from build123d import *

# Parameters (mm, degrees)
ESBO_O1_R             = 75
ESBO_O1_R_2           = 8.5
EXTRUS_O1_DEPTH       = 3.35
ESBO_O2_R             = 24.25
CORTE_EXTRUS_O1_DEPTH = 1
CORTE_EXTRUS_O3_DEPTH = 10
LPATTERN3_COUNT       = 2
LPATTERN3_PITCH       = 28
FILETE1_R             = 2


with BuildPart() as part:
    # Esboço1 → Extrusão1 (new body)
    with BuildSketch(Plane.XY):
        Circle(ESBO_O1_R)
        Circle(ESBO_O1_R_2, mode=Mode.SUBTRACT)
    extrude(amount=EXTRUS_O1_DEPTH)

    # Esboço2 → Corte-extrusão1 (cut)
    with BuildSketch(Plane(origin=(0, 0, 0), x_dir=(-1, 0, 0), z_dir=(0, 0, -1))):
        Circle(ESBO_O2_R)
    extrude(amount=-CORTE_EXTRUS_O1_DEPTH, mode=Mode.SUBTRACT)

    # Esboço6 → Corte-extrusão3 (cut)
    with BuildSketch(Plane(origin=(0, 0, 0), x_dir=(-1, 0, 0), z_dir=(0, 0, -1))):
        with BuildLine():
            Line((-5, 25.5), (5, 25.5))
            ThreePointArc((5, 25.5), (7.5, 28), (5, 30.5))
            Line((5, 30.5), (-5, 30.5))
            ThreePointArc((-5, 30.5), (-7.5, 28), (-5, 25.5))
        make_face()
    extrude(amount=-CORTE_EXTRUS_O3_DEPTH, mode=Mode.SUBTRACT)

    # Esboço8 → Escareado para SFHCS M63 (revolve, cut)
    with BuildSketch(Plane(origin=(17.5, 33.25, 0), x_dir=(0, 1, 0), z_dir=(1, 0, 0))):
        Polygon((0, 0), (0, 3.35), (3.3, 3.35), (3.3, 3.42), (6.72, 0), align=None)
    escareado_para_sfhcs_m63 = revolve(axis=Axis((17.5, 33.25, -6.35), (0, 0, 1)), mode=Mode.SUBTRACT)

    # LPattern3: Escareado para SFHCS M63 ×2
    with Locations(*[(i * LPATTERN3_PITCH, 0, 0) for i in range(1, LPATTERN3_COUNT)]):
        add(escareado_para_sfhcs_m63, mode=Mode.SUBTRACT)

    # Filete1
    filete1_edges = [part.edges().sort_by_distance(p)[0] for p in [
        (-75, 0, 0),
    ]]
    fillet(filete1_edges, radius=FILETE1_R)


solid = part.part
Work out the finished part from the listing and answer in its coordinate system (mm). A direction names the side the tool comes from. Give positions to 0.01 mm unless a question says otherwise; leave off trailing zeros. Order: outer loops, then holes, each group sorted by start corner. A loop starts at its lowest first (then second) coordinate and runs counter-clockwise, first axis right, second up. Notation, with made-up numbers: (-23.75, -18.75) -> (-7.75, -18.75) arc R19 cw to (-7.75, -14.75) -> close; hole circle Ø6 at (62.25, -21.5). An arc over 180 degrees is marked (long way). Answer as a JSON object with one key per item and string values. Group by question number.
1. Section A-A on x = 0 is taken. Determine the outline of the cut face in (y, z), plus the area to 3 significant figures.
2. The mould has two halves that part along Y. Classify faces 1 (the flat face through (-10, 0, 1)), 2 (the cylindrical face through (-9.764, 74.362, 2.666)), 3 (the flat face through (-1, -31, 0)): released by +Y, released by -Y, zero draft, split by the parting line, or undercut.
3. A tool of negligible diameter and unlimited length cuts with its end or side. For faces 4 (the flat face through (0, 25.5, 2)), 5 (the cylindrical face through (-11.19, -21.514, 0.493)), 6 (the flat face through (-1, -16, 3.35)), from which of +Z, -Z, +X, -X, +Y, -Y can it reach the whole face along a straight path? Write none if from no direction.
4. Section B-B on y = 0 is taken. Determine the outline of the cut face in (x, z).
5. Flat-ended cylindrical pins translate along their axes: pin 1 Ø4 at (x, y) = (-26, 37) entering from -Z; pin 2 Ø1 at (x, z) = (31, 0.5) entering from +Y; pin 3 Ø1.5 at (y, z) = (55, 2.5) entering from -X; pin 4 Ø22 at (x, y) = (0, 0) entering from -Z. Find the tip coordinate at first contact, or state that the pin passes through.
6. Consider line 1 along Y through (x, z) = (0, 2.35); line 2 along Y through (x, z) = (0, 0.55); line 3 along X through (y, z) = (-17, 2.4). Determine where each line is inside the solid, lowest interval first. Write a range as [from, to].
Result sheet:
{
 "1": {"outline": "(-75, 2) arc R2 ccw to (-73, 0) -> (-24.25, 0) -> (-24.25, 1) -> (-8.5, 1) -> (-8.5, 3.35) -> (-75, 3.35) -> close; (8.5, 1) -> (24.25, 1) -> (24.25, 0) -> (25.5, 0) -> (25.5, 3.35) -> (8.5, 3.35) -> close; (30.5, 0) -> (73, 0) arc R2 ccw to (75, 2) -> (75, 3.35) -> (30.5, 3.35) -> close", "area": "396 mm^2"},
 "2": {"face 1": "undercut", "face 2": "split by the parting line", "face 3": "zero draft"},
 "3": {"face 4": "+Z, -Z", "face 5": "-Z", "face 6": "+Z, +X, -X, +Y, -Y"},
 "4": {"outline": "(-75, 2) arc R2 ccw to (-73, 0) -> (-24.25, 0) -> (-24.25, 1) -> (-8.5, 1) -> (-8.5, 3.35) -> (-75, 3.35) -> close; (8.5, 1) -> (24.25, 1) -> (24.25, 0) -> (73, 0) arc R2 ccw to (75, 2) -> (75, 3.35) -> (8.5, 3.35) -> close"},
 "5": {"pin 1": "stops at z = 0", "pin 2": "stops at y = 68.07", "pin 3": "stops at x = -51.79", "pin 4": "stops at z = 1"},
 "6": {"line 1": "y = [-75, -8.5], [8.5, 25.5], [30.5, 75]", "line 2": "y = [-74.38, -24.25], [24.25, 25.5], [30.5, 74.38]", "line 3": "x = [-73.05, 73.05]"}
}
